Part print with two shaded views. Sizes in mm from the minimum x, y, z corner. Coordinates: 2 decimals unless noted, no trailing zeros. Order: outer loops, then holes, each group sorted by start corner. A loop starts at its lowest first (then second) coordinate and runs counter-clockwise, first axis right, second up.
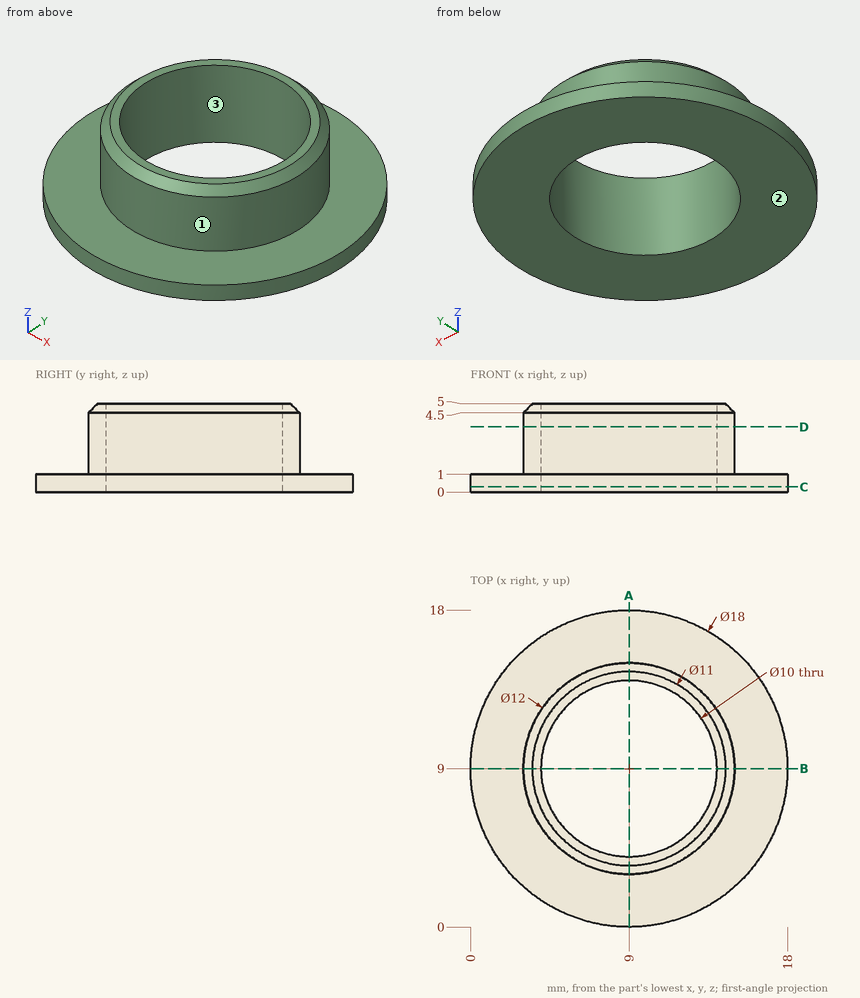
Q1. Cut at C-C on z = 0.3. Write the cut outline in (x, y), and give its area (3 significant figures).
Results list:
outline: circle Ø18 at (9, 9); hole circle Ø10 at (9, 9)
area: 176 mm2
Q2. Mould opens along X. For the marked faces 1, 2 and 3 say: pulls with the +X half, pulls with the -X half, needs draft (parallel to the pull), parting line crosses it, or undercut.
Results list:
face 1: parting line crosses it
face 2: needs draft
face 3: undercut
Q3. Pin check, flat tips, straight feed: pin 1 Ø8 at (x, y) = (16, 11.5) entering from -Z; pin 2 Ø1.5 at (x, y) = (3, 5) entering from +Z; pin 3 Ø1 at (y, z) = (3.5, 3.5) entering from +X. Stop position of each tip, or through.
Results list:
pin 1: stops at z = 0
pin 2: stops at z = 1
pin 3: stops at x = 12.32
Q4. Cut at D-D on z = 3.7. Write the cut outline in (x, y), and give its area (3 significant figures).
Results list:
outline: circle Ø12 at (9, 9); hole circle Ø10 at (9, 9)
area: 34.6 mm2
Q5. Cut at A-A on x = 9. Write the cut outline in (y, z), and give its area (4 significant figures).
Results list:
outline: (0, 0) - (4, 0) - (4, 5) - (3.5, 5) - (3, 4.5) - (3, 1) - (0, 1) - close; (14, 0) - (18, 0) - (18, 1) - (15, 1) - (15, 4.5) - (14.5, 5) - (14, 5) - close
area: 15.75 mm2
Q6. Wall check: line 1 along Y through (x, z) = (9, 2.25); line 2 along Z through (x, y) = (17, 13); line 3 along X through (y, z) = (12.75, 2.6). Give the ranges that are in metal, low to high.
Results list:
line 1: y = 3 to 4, 14 to 15
line 2: z = 0 to 1
line 3: x = 4.32 to 5.69, 12.31 to 13.68
